```python
from build123d import *

# Parameters (mm, degrees)
F0_W     = 60
F0_H     = 60
F1_DEPTH = 9
F4_DEPTH = 25
F5_DEPTH = 50
F6_DEPTH = 55
F7_DEPTH = 25
F9_D     = 50


with BuildPart() as f1:
    # F0 (on Top) → F1 (new body)
    with BuildSketch(Plane.XY):
        with Locations((16.955535, 22.425423)):
            Rectangle(F0_W, F0_H)
    extrude(amount=F1_DEPTH)

    # F2 (on Right) → F4 (cut)
    with BuildSketch(Plane.YZ):
        Polygon((-7.574577, 9), (-7.574577, 0), (-6.036178, 9), align=None)
        Polygon((50.887025, 9), (52.425423, 0), (52.425423, 9), align=None)
    extrude(amount=-F4_DEPTH, mode=Mode.SUBTRACT)

    # F2 (on Right) → F5 (cut)
    with BuildSketch(Plane.YZ):
        Polygon((-7.574577, 9), (-7.574577, 0), (-6.036178, 9), align=None)
        Polygon((50.887025, 9), (52.425423, 0), (52.425423, 9), align=None)
    extrude(amount=F5_DEPTH, mode=Mode.SUBTRACT)

    # F3 (on Front) → F6 (cut)
    with BuildSketch(Plane.XZ):
        Polygon((-13.044465, 9), (-13.044465, 0), (-11.506067, 9), align=None)
        Polygon((45.417137, 9), (46.955535, 0), (46.955535, 9), align=None)
    extrude(amount=-F6_DEPTH, mode=Mode.SUBTRACT)

    # F3 (on Front) → F7 (cut)
    with BuildSketch(Plane.XZ):
        Polygon((-13.044465, 9), (-13.044465, 0), (-11.506067, 9), align=None)
        Polygon((45.417137, 9), (46.955535, 0), (46.955535, 9), align=None)
    extrude(amount=F7_DEPTH, mode=Mode.SUBTRACT)

    # F9 (through all)
    with Locations(Plane.XY.offset(9)):
        with Locations((16.955535, 22.425423)):
            Hole(F9_D / 2)


solid = f1.part
```
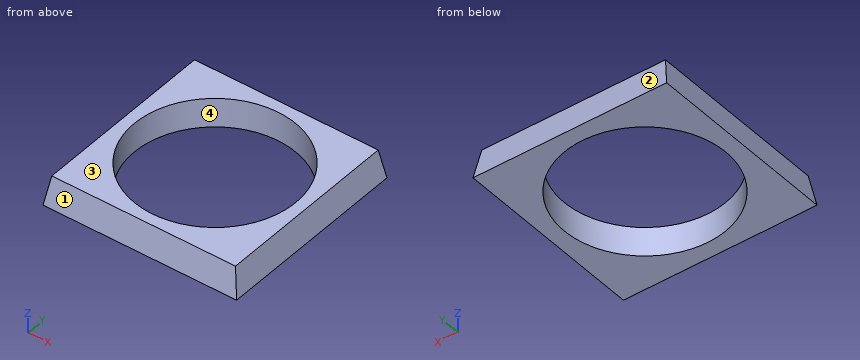
Geometry check sheet. Reference: the model listing, model coordinates, mm. Face numbers are marked on the shaded views. Coordinates: 2 decimals unless noted, no trailing zeros. Write each loop counter-clockwise with the first axis right and the second up, starting at its lowest first coordinate (ties: lowest second). Pieces come first, ordered by that corner, then holes. Notation, with made-up numbers: M -28,35.5 L 12,35.5 A19 ccw 12,72.5 Z; hole C 50.5,25 d4. An arc over 180 degrees is marked long. Answer as a JSON object with one key per item and string values.
1. Section check B-B, the plane x = 41. Enter the section's corners in (y, z), plus the area to 3 significant figures.
Answers below:
{"outline": "M -7.57,0 L 15.58,0 L 15.58,9 L -6.04,9 Z; M 29.27,0 L 52.43,0 L 50.89,9 L 29.27,9 Z", "area": "403 mm²"}
2. Scan lines: L1, parallel to X at y = 44, z = 8.25; L2, parallel to X at y = 41, z = 6.5; L3, parallel to Y at x = 8, z = 4.5. Record each from-to range of solid material in increasing order.
Answers below:
{"L1": "x = -11.63 to 4.32, 29.59 to 45.55", "L2": "x = -11.93 to 0.22, 33.69 to 45.84", "L3": "y = -6.81 to -0.92, 45.77 to 51.66"}
3. Go/stop test with flat-tipped pins: pin 1 Ø1 at (y, z) = (17.5, 7) entering from -X; pin 2 Ø2 at (x, z) = (10, 1.5) entering from +Y; pin 3 Ø5 at (y, z) = (13.5, 4.5) entering from +X. Record where each tip stops, or that it passes through.
Answers below:
{"pin 1": "stops at x = -11.93", "pin 2": "stops at y = 52.34", "pin 3": "stops at x = 46.61"}
4. Section check C-C, the plane z = 4. Enter the section's corners in (x, y).
Answers below:
{"outline": "M -12.36,-6.89 L 46.27,-6.89 L 46.27,51.74 L -12.36,51.74 Z; hole C 16.96,22.43 d50"}
5. Section check A-A, the plane y = 30.5. Enter the section's corners in (x, z), plus the area to 3 significant figures.
Answers below:
{"outline": "M -13.04,0 L -6.7,0 L -6.7,9 L -11.51,9 Z; M 40.62,0 L 46.96,0 L 45.42,9 L 40.62,9 Z", "area": "100 mm²"}
6. Section check D-D, the plane y = 48.5. Enter the section's corners in (x, z).
Answers below:
{"outline": "M -13.04,0 L 46.96,0 L 45.42,9 L -11.51,9 Z"}
7. Draft check along Y on the marked faces 1, 2, 3 and 4. Enter one of: released by +Y, released by -Y, zero draft, split by the parting line, or undercut.
Answers below:
{"face 1": "released by -Y", "face 2": "released by +Y", "face 3": "zero draft", "face 4": "undercut"}
